Autodesk Inventor part; units mm, degrees
ref_plane "YZ Plane" through (0, 0, 0) normal (1, 0, 0) x (0, 1, 0)
ref_plane "XZ Plane" through (0, 0, 0) normal (0, 1, 0) x (-1, 0, 0)
ref_plane "XY Plane" through (0, 0, 0) normal (0, 0, 1) x (1, 0, 0)
sketch "Sketch1" plane through (0, 0, 0) normal (0, 1, 0) x (-1, 0, 0)
  line L0 (-44.2289, 0) -> (-44.2289, -28.14)
  line L1 (-0.4496, -28.14) -> (-0.4496, 0)
  circle A0 centre (23.79, -17.595) radius 1.05
  circle A1 centre (23.79, -2.545) radius 1.05
  circle A2 centre (8.69, -17.595) radius 1.05
  circle A3 centre (8.69, -2.545) radius 1.05
  circle A4 centre (-53.5486, -10.07) radius 1.05
  circle A5 centre (-60.8486, -17.07) radius 1.05
  circle A6 centre (-60.8486, -3.07) radius 1.05
  circle A7 centre (-74.0686, -18.07) radius 1.05
  circle A8 centre (-74.0686, -2.07) radius 1.05
  circle A9 centre (-37.3393, -39.96) radius 1.55
  circle A10 centre (-22.3393, -39.96) radius 1.55
  circle A11 centre (-7.3393, -39.96) radius 1.55
  arc A12 (35.49, -3.3676) -> (35.49, -16.7724) centre (36.29, -10.07) ccw
  line L2 (35.49, -1) -> (35.49, -3.3676)
  arc A13 (-80.1686, -16.7724) -> (-80.1686, -3.3676) centre (-80.9686, -10.07) ccw
  line L3 (-80.1686, -27.14) -> (-80.1686, -16.7724)
  arc A14 (-80.1686, -27.14) -> (-79.1686, -28.14) centre (-79.1686, -27.14) ccw
  line L4 (-43.7793, -28.14) -> (-79.1686, -28.14)
  line L5 (-43.7793, -50) -> (-43.7793, -28.14)
  line L6 (-0.8993, -50) -> (-43.7793, -50)
  line L7 (-0.8993, -28.14) -> (-0.8993, -50)
  line L8 (34.49, -28.14) -> (-0.8993, -28.14)
  arc A15 (34.49, -28.14) -> (35.49, -27.14) centre (34.49, -27.14) ccw
  line L9 (35.49, -16.7724) -> (35.49, -27.14)
  arc A16 (35.49, -1) -> (34.49, 0) centre (34.49, -1) ccw
  line L10 (-79.1686, 0) -> (34.49, 0)
  arc A17 (-79.1686, 0) -> (-80.1686, -1) centre (-79.1686, -1) ccw
  line L11 (-80.1686, -3.3676) -> (-80.1686, -1)
  line L12 (-44.6786, -28.14) -> (-44.6786, 0)
  line L13 (-43.7793, 0) -> (-43.7793, -28.14)
  line L14 (-0.8993, -28.14) -> (-0.8993, 0)
  line L15 (0, 0) -> (0, -28.14)
extrude "Extrusion1" add sketch "Sketch1" against normal blind 1.5
properties part number "axis_22_top_frame"
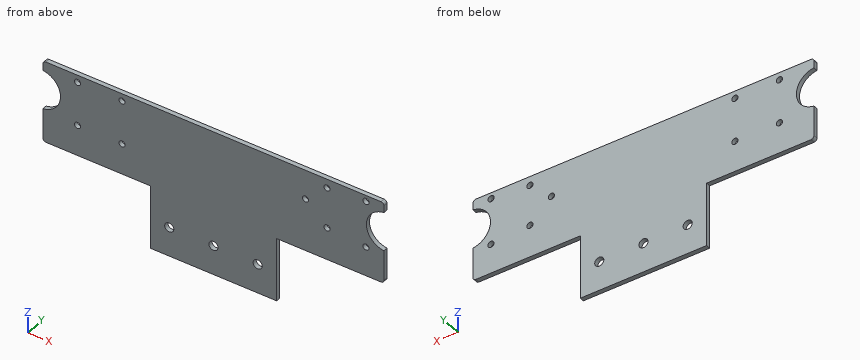
Work out the finished part from the listing and answer in its coordinate system (mm). Coordinates: 2 decimals unless noted, no trailing zeros. Order: outer loops, then holes, each group sorted by start corner. A loop starts at its lowest first (then second) coordinate and runs counter-clockwise, first axis right, second up. Notation, with made-up numbers: (59, -14) - (98, -14) arc R15 ccw to (98, -1) - close; hole circle Ø6 at (-2.5, -27.75). An arc over 180 degrees is marked (long way). Answer as a JSON object with one key per item and string values.
1. This flat-tipped pin is pushed along its axis until it touches: P1, Ø0.8, axis at y = -0.5, z = -37, coming from the -X side. Where does it stop, or does it pass through?
Output values:
{"P1": "stops at x = 0.9"}
2. Find section B-B on z = -39.96. Determine the outline of the cut face in (x, y).
Output values:
{"outline": "(0.9, -1.5) - (5.79, -1.5) - (5.79, 0) - (0.9, 0) - close; (8.89, -1.5) - (20.79, -1.5) - (20.79, 0) - (8.89, 0) - close; (23.89, -1.5) - (35.79, -1.5) - (35.79, 0) - (23.89, 0) - close; (38.89, -1.5) - (43.78, -1.5) - (43.78, 0) - (38.89, 0) - close"}
3. Find section A-A on x = -8.69. Determine the outline of the cut face in (y, z) (3 decimals), plus the area to 3 significant figures.
Output values:
{"outline": "(-1.5, -28.14) - (0, -28.14) - (0, -18.645) - (-1.5, -18.645) - close; (-1.5, -16.545) - (0, -16.545) - (0, -3.595) - (-1.5, -3.595) - close; (-1.5, -1.495) - (0, -1.495) - (0, 0) - (-1.5, 0) - close", "area": "35.9 mm²"}
4. Find section D-D on y = -0.6. Count the separate pieces of the cut face and the enclosed holes in it, plus the area to 3 significant figures.
Output values:
{"separate pieces": "1", "enclosed holes": "12", "area": "4,020 mm²"}
5. Find section C-C on x = 37.5. Determine the outline of the cut face in (y, z), plus the area to 3 significant figures.
Output values:
{"outline": "(-1.5, -50) - (0, -50) - (0, -41.5) - (-1.5, -41.5) - close; (-1.5, -38.42) - (0, -38.42) - (0, 0) - (-1.5, 0) - close", "area": "70.4 mm²"}
6. Consider line 1 (Z direction, x = -8.69, y = -0.35) (3 decimals); line 2 (Z direction, x = 47, y = -1.05); line 3 (X direction, y = -0.2, z = -47). Determine where each line is inside the solid, lowest interval first.
Output values:
{"line 1": "z = -28.14 to -18.645, -16.545 to -3.595, -1.495 to 0", "line 2": "z = -28.14 to 0", "line 3": "x = 0.9 to 43.78"}
